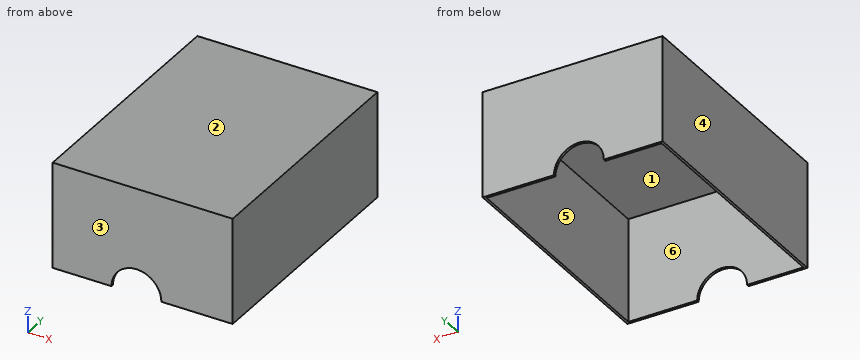
Autodesk Inventor part; units mm, degrees
ref_plane "Arbeitsebene2" through (-34.54, -42.79, -40) normal (0, 0, 1) x (1, 0, 0)
ref_plane "Arbeitsebene3" through (-32.5, -40, -41) normal (0, 0, -1) x (0, 1, 0)
ref_plane "YZ Plane" through (0, 0, 0) normal (1, 0, 0) x (0, 1, 0)
ref_plane "Arbeitsebene1" through (0, 0, 0.5) normal (0, 0, 1) x (1, 0, 0)
sketch "Skizze1" plane through (0, 0, 0.5) normal (0, 0, 1) x (1, 0, 0)
  line L0 (-33.9, -46.4) -> (-33.9, 46.4)
  line L1 (-33.9, 46.4) -> (33.9, 46.4)
  line L2 (33.9, 46.4) -> (33.9, -46.4)
  line L3 (33.9, -46.4) -> (-33.9, -46.4)
  line L4 (35, 47.5) -> (-35, 47.5)
  line L5 (-35, 47.5) -> (-35, -47.5)
  line L6 (-35, -47.5) -> (35, -47.5)
  line L7 (35, -47.5) -> (35, 47.5)
  line L8 (-36.1, 48.6) -> (36.1, 48.6)
  line L9 (36.1, 48.6) -> (36.1, -48.6)
  line L10 (36.1, -48.6) -> (-36.1, -48.6)
  line L11 (-36.1, -48.6) -> (-36.1, 48.6)
  point P0 (0, 0)
  dimension "d0" = 1.1
extrude "Extrusion1" add sketch "Skizze1" along normal blind 1 contours L0 L1 L2 L3 | L7 L6 L5 L4 | L8 L9 L10 L11
sketch "Skizze2" plane through (0, 0, 0.5) normal (0, 0, -1) x (-1, 0, 0)
  line L0 (36.1, 48.6) -> (-36.1, 48.6)
  line L1 (-36.1, 48.6) -> (-36.1, -48.6)
  line L2 (-36.1, -48.6) -> (36.1, -48.6)
  line L3 (36.1, -48.6) -> (36.1, 48.6)
  line L4 (-35.1, 47.6) -> (35.1, 47.6)
  line L5 (35.1, 47.6) -> (35.1, -47.6)
  line L6 (35.1, -47.6) -> (-35.1, -47.6)
  line L7 (-35.1, -47.6) -> (-35.1, 47.6)
  point P0 (0, 0)
  dimension "d3" = 1
ref_plane "Arbeitsebene2" through (-34.54, -42.79, -40) normal (0, 0, 1) x (1, 0, 0)
ref_plane "Arbeitsebene3" through (-32.5, -40, -41) normal (0, 0, -1) x (0, 1, 0)
extrude "Extrusion2" add sketch "Skizze2" along normal up to surface (41.5 mm away)
sketch "Skizze3" plane through (-36.1, -48.6, 1.5) normal (0, -1, 0) x (1, 0, 0)
  line L0 (0, -42.5) -> (72.2, -42.5)
  line L1 (33.6, -45.4928) -> (33.6, 6) construction
  circle A0 centre (33.6, -42.5) radius 10
  point P0 (36.1, -1.5)
  dimension "d6" = 20
extrude "Extrusion3" cut sketch "Skizze3" against normal up to surface (97.2 mm away)
properties part number "Deckel"
Check sheet for the modelled part. Datum: model origin and axes. Units: mm. Face numbers are marked on the shaded views. A direction names the side the tool comes from. Round coordinates to 2 decimals unless told otherwise and drop trailing zeros. Loops run counter-clockwise (first coordinate to the right, second up) from the corner with the lowest first, then second, coordinate; pieces in that order, holes last. Notation, with made-up numbers: M -18.5,-29 L 21.5,-29 A36 ccw 21.5,8 Z; hole C 71,87.5 d1. An arc over 180 degrees is marked long. One line per question, with ' | ' between items. Start each with the question number.
Item 1: Scan lines: probe 1 along Y at (x, z) = (20.5, -8); probe 2 along X at (y, z) = (27, -37); probe 3 along Z at (x, y) = (-11, 42). Record each from-to range of solid material in increasing order.
Item 2: Release check for a two-part mould opening along Y. For the marked faces 3, 4, 5 and 6 record: released by +Y, released by -Y, zero draft, split by the parting line, or undercut.
Item 3: Section check B-B (y = -5). Record the boundary of the cut face in (x, z), and give its area (3 significant figures).
Item 4: Section check A-A (z = -7.5). Record the boundary of the cut face in (x, y), and give its area (3 significant figures).
Item 5: Set-up check for the marked faces 1 and 2: record each of +Z, -Z, +X, -X, +Y, -Y from which the full face is reachable in a straight line by a thin tool's end or side.
Item 6: Gauge pin test, flat end, axial feed: pin 1 Ø12 at (x, y) = (-7.5, 21) entering from -Z. Record the tip position at first contact, or that the pin passes through.
Item 7: Section check C-C (x = -24.5). Record the boundary of the cut face in (y, z).
Worked out:
1) probe 1: -48.6 to -47.6, 47.6 to 48.6 | probe 2: -36.1 to -35.1, 35.1 to 36.1 | probe 3: 0.5 to 1.5
2) face 3: released by -Y | face 4: zero draft | face 5: undercut | face 6: undercut
3) outline: M -36.1,-41 L -35.1,-41 L -35.1,0.5 L 35.1,0.5 L 35.1,-41 L 36.1,-41 L 36.1,1.5 L -36.1,1.5 Z | area: 155 mm^2
4) outline: M -36.1,-48.6 L 36.1,-48.6 L 36.1,48.6 L -36.1,48.6 Z; hole M -35.1,-47.6 L 35.1,-47.6 L 35.1,47.6 L -35.1,47.6 Z | area: 335 mm^2
5) face 1: -Z | face 2: +Z, +X, -X, +Y, -Y
6) pin 1: z = 0.5
7) outline: M -48.6,-41 L -47.6,-41 L -47.6,0.5 L 47.6,0.5 L 47.6,-41 L 48.6,-41 L 48.6,1.5 L -48.6,1.5 Z
